Work out the finished part from the listing and answer in its coordinate system (mm). Face numbers are marked on the shaded views. A direction names the side the tool comes from. Round coordinates to 2 decimals unless told otherwise and drop trailing zeros. Write each loop counter-clockwise with the first axis right and the second up, starting at its lowest first coordinate (ties: lowest second). Pieces come first, ordered by that corner, then holes. Notation, with made-up numbers: (60, 71.5) - (119, 71.5) arc R32 ccw to (119, 101.5) - close; hole circle Ø3 at (-23, 19.5). An arc over 180 degrees is marked (long way). Answer as a JSON object with one key per item and string values.
```python
from build123d import *

# Parameters (mm, degrees)
EXTRUDE_1_DEPTH     = 10
SKETCH_2_R          = 2.5
CUT_EXTRUDE_1_DEPTH = 10
SKETCH_3_R          = 2.5
CUT_EXTRUDE_2_DEPTH = 10


with BuildPart() as part:
    # 草图1 → 凸台-拉伸1 (new body)
    with BuildSketch(Plane.XY):
        Polygon((0, 0), (13, 0), (13, -2), (-2, -2), (-2, 13), (0, 13), align=None)
    extrude(amount=EXTRUDE_1_DEPTH)

    # 草图2 → 切除-拉伸1 (cut)
    with BuildSketch(Plane.XZ.offset(2)):
        with Locations((5.5, 5)):
            Circle(SKETCH_2_R)
    extrude(amount=-CUT_EXTRUDE_1_DEPTH, mode=Mode.SUBTRACT)

    # 草图3 → 切除-拉伸2 (cut)
    with BuildSketch(Plane.ZY.offset(2)):
        with Locations((5, 5.5)):
            Circle(SKETCH_3_R)
    extrude(amount=-CUT_EXTRUDE_2_DEPTH, mode=Mode.SUBTRACT)


solid = part.part
```
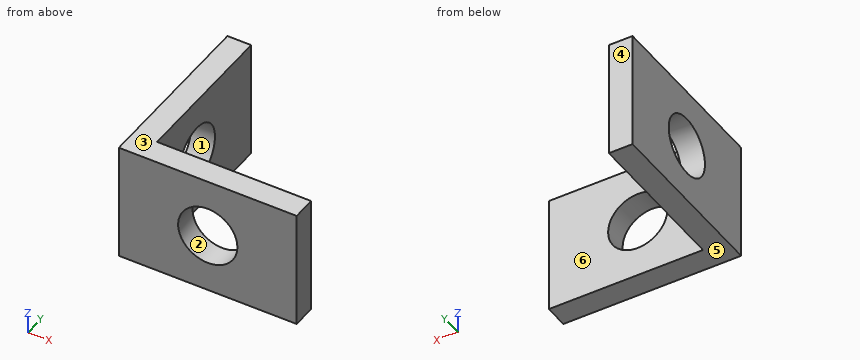
Item 1: For the marked faces 5 and 6, determine the directions among +Z, -Z, +X, -X, +Y, -Y from which every point of the face is accessible in a straight line to the end or side of a thin tool.
Results found:
{"face 5": "-Z, +X, -X, +Y, -Y", "face 6": "+Z, -Z, +X, +Y"}
Item 2: Determine the mould class of the marked faces 1, 2, 3 and 4 for opening direction Z: pulls with the +Z half, pulls with the -Z half, needs draft (parallel to the pull), parting line crosses it, or undercut.
Results found:
{"face 1": "undercut", "face 2": "undercut", "face 3": "pulls with the +Z half", "face 4": "needs draft"}
Item 3: Each of these flat-tipped pins is pushed along its axis until it touches: P1, Ø1.5, axis at x = 7.5, z = 8.5, coming from the +Y side; P2, Ø4.5, axis at y = 5.5, z = 5, coming from the +X side. Where does it stop, or does it pass through?
Results found:
{"P1": "y = 0", "P2": "through"}
Item 4: A cutting plane is placed at D-D (y = -0.5). Write down the section's boundary in (x, z).
Results found:
{"outline": "(-2, 0) - (13, 0) - (13, 10) - (-2, 10) - close; hole circle Ø5 at (5.5, 5)"}
Item 5: A cutting plane is placed at A-A (z = 6.5). Write down the section's boundary in (x, y).
Results found:
{"outline": "(-2, -2) - (3.5, -2) - (3.5, 0) - (0, 0) - (0, 3.5) - (-2, 3.5) - close; (-2, 7.5) - (0, 7.5) - (0, 13) - (-2, 13) - close; (7.5, -2) - (13, -2) - (13, 0) - (7.5, 0) - close"}
Item 6: Consider line 1 along Z through (x, y) = (5.5, -1.25); line 2 along Y through (x, z) = (-1.5, 5); line 3 along Y through (x, z) = (1.75, 2.25). Determine where each line is inside the solid, lowest interval first.
Results found:
{"line 1": "0 to 2.5, 7.5 to 10", "line 2": "-2 to 3, 8 to 13", "line 3": "-2 to 0"}
Item 7: A cutting plane is placed at C-C (y = 4). Write down the section's boundary in (x, z), and give its area (3 significant figures).
Results found:
{"outline": "(-2, 0) - (0, 0) - (0, 3) - (-2, 3) - close; (-2, 7) - (0, 7) - (0, 10) - (-2, 10) - close", "area": "12.0 mm²"}
Item 8: A cutting plane is placed at B-B (x = 7.5). Write down the section's boundary in (y, z), and give its area (3 significant figures).
Results found:
{"outline": "(-2, 0) - (0, 0) - (0, 3.5) - (-2, 3.5) - close; (-2, 6.5) - (0, 6.5) - (0, 10) - (-2, 10) - close", "area": "14.0 mm²"}
